from build123d import *

# Parameters (mm, degrees)
F0_W     = 330
F0_H     = 33.8
F1_DEPTH = 21.2
F2_R     = 1.395
F3_DEPTH = 10
F4_R     = 1.75
F5_DEPTH = 11.3


with BuildPart() as f1:
    # F0 (on Top) → F1 (new body)
    with BuildSketch(Plane.XY):
        with Locations((95, 0)):
            Rectangle(F0_W, F0_H)
    extrude(amount=F1_DEPTH)

    # F2 (on face) → F3 (cut)
    with BuildSketch(Plane(origin=(0, 0, 0), x_dir=(1, 0, 0), z_dir=(0, 0, -1))):
        Circle(F2_R)
        with Locations((190, 0)):
            Circle(F2_R)
    extrude(amount=-F3_DEPTH, mode=Mode.SUBTRACT)

    # F4 (on face) → F5 (join)
    with BuildSketch(Plane.XY.offset(21.2)):
        with Locations((-57, 8.5)):
            Circle(F4_R)
        with Locations((-57, -8.5)):
            Circle(F4_R)
        with Locations((-48, 0)):
            Circle(F4_R)
        with Locations((-39, 8.5)):
            Circle(F4_R)
        with Locations((-39, -8.5)):
            Circle(F4_R)
        with Locations((-30, 0)):
            Circle(F4_R)
        with Locations((-21, 8.5)):
            Circle(F4_R)
        with Locations((-21, -8.5)):
            Circle(F4_R)
        with Locations((-12, 0)):
            Circle(F4_R)
        with Locations((-3, 8.5)):
            Circle(F4_R)
        with Locations((-3, -8.5)):
            Circle(F4_R)
        with Locations((6, 0)):
            Circle(F4_R)
        with Locations((15, 8.5)):
            Circle(F4_R)
        with Locations((15, -8.5)):
            Circle(F4_R)
        with Locations((24, 0)):
            Circle(F4_R)
        with Locations((33, 8.5)):
            Circle(F4_R)
        with Locations((33, -8.5)):
            Circle(F4_R)
        with Locations((42, 0)):
            Circle(F4_R)
        with Locations((51, 8.5)):
            Circle(F4_R)
        with Locations((51, -8.5)):
            Circle(F4_R)
        with Locations((60, 0)):
            Circle(F4_R)
        with Locations((69, 8.5)):
            Circle(F4_R)
        with Locations((69, -8.5)):
            Circle(F4_R)
        with Locations((78, 0)):
            Circle(F4_R)
        with Locations((87, 8.5)):
            Circle(F4_R)
        with Locations((87, -8.5)):
            Circle(F4_R)
        with Locations((96, 0)):
            Circle(F4_R)
        with Locations((105, 8.5)):
            Circle(F4_R)
        with Locations((105, -8.5)):
            Circle(F4_R)
        with Locations((114, 0)):
            Circle(F4_R)
        with Locations((123, 8.5)):
            Circle(F4_R)
        with Locations((123, -8.5)):
            Circle(F4_R)
        with Locations((132, 0)):
            Circle(F4_R)
        with Locations((141, 8.5)):
            Circle(F4_R)
        with Locations((141, -8.5)):
            Circle(F4_R)
        with Locations((150, 0)):
            Circle(F4_R)
        with Locations((159, 8.5)):
            Circle(F4_R)
        with Locations((159, -8.5)):
            Circle(F4_R)
        with Locations((168, 0)):
            Circle(F4_R)
        with Locations((177, 8.5)):
            Circle(F4_R)
        with Locations((177, -8.5)):
            Circle(F4_R)
        with Locations((186, 0)):
            Circle(F4_R)
        with Locations((195, 8.5)):
            Circle(F4_R)
        with Locations((195, -8.5)):
            Circle(F4_R)
        with Locations((204, 0)):
            Circle(F4_R)
        with Locations((213, 8.5)):
            Circle(F4_R)
        with Locations((213, -8.5)):
            Circle(F4_R)
        with Locations((222, 0)):
            Circle(F4_R)
        with Locations((231, 8.5)):
            Circle(F4_R)
        with Locations((231, -8.5)):
            Circle(F4_R)
        with Locations((240, 0)):
            Circle(F4_R)
        with Locations((249, 8.5)):
            Circle(F4_R)
        with Locations((249, -8.5)):
            Circle(F4_R)
    extrude(amount=F5_DEPTH)


solid = f1.part
Can you work these out from the model? Positions are in its coordinate system, mm. Give positions to 0.01 mm unless a question says otherwise; leave off trailing zeros. Use one line per item in the form item = value.
1) We'd pull the mould along X, two halves only. Please class faces 1 (the face through (93, 16.9, 10)), 2 (the face through (93, 0, 21.2)), 3 (the face through (-70, 0, 10)): released by +X, released by -X, zero draft, split by the parting line, or undercut.
Answers:
face_1 = zero draft
face_2 = undercut
face_3 = released by -X
2) Will this pin go through, and if not, where does the flat tip stop? pin 1 (4 mm diameter, centred on x = 50, y = -0.5, fed in from +Z).
Answers:
pin_1 = 21.2
3) If we section it at A-A (z = 29.5): Count the separate pieces of the cut face and the enclosed holes in it, plus the area to 3 significant figures.
Answers:
separate_pieces = 53
enclosed_holes = 0
area = 510 mm²
4) I need wall thicknesses on line 1 along X through (y, z) = (0, 5.25) (3 decimals); line 2 along Y through (x, z) = (0, 7) (3 decimals); line 3 along Y through (x, z) = (195, 22). Which ranges of each line are inside material? Lowest first, please.
Answers:
line_1 = -70 to -1.395, 1.395 to 188.605, 191.395 to 260
line_2 = -16.9 to -1.395, 1.395 to 16.9
line_3 = -10.25 to -6.75, 6.75 to 10.25
